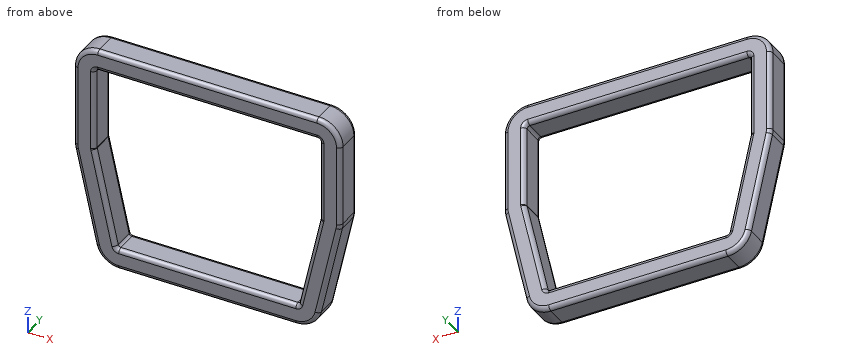
Autodesk Inventor part; units mm, degrees
ref_plane "YZ Plane" through (0, 0, 0) normal (1, 0, 0) x (0, 1, 0)
ref_plane "XZ Plane" through (0, 0, 0) normal (0, 1, 0) x (-1, 0, 0)
ref_plane "XY Plane" through (0, 0, 0) normal (0, 0, 1) x (1, 0, 0)
sketch "Sketch1" plane through (0, 0, 0) normal (0, 1, 0) x (-1, 0, 0)
  line L0 (-7.8, 0) -> (7.8, 0)
  arc A0 (8, -0.2) -> (7.8, 0) centre (7.8, -0.2) ccw
  arc A1 (-7.8, 0) -> (-8, -0.2) centre (-7.8, -0.2) ccw
  line L1 (-8, -0.2) -> (-8, -6)
  line L2 (8, -0.2) -> (8, -6)
  arc A2 (-8, -6) -> (-7.9953, -6.043) centre (-7.8, -6) ccw
  arc A3 (7.9953, -6.043) -> (8, -6) centre (7.8, -6) ccw
  line L3 (-7.9953, -6.043) -> (-6.5, -12.843)
  line L4 (7.9953, -6.043) -> (6.5, -12.843)
  arc A4 (-6.5, -12.843) -> (-6.3047, -13) centre (-6.3047, -12.8) ccw
  line L5 (-6.3047, -13) -> (6.3047, -13)
  arc A5 (6.3047, -13) -> (6.5, -12.843) centre (6.3047, -12.8) ccw
  line L6 (-9.5, -6) -> (-9.5, -0.2)
  arc A6 (-7.8, 1.5) -> (-9.5, -0.2) centre (-7.8, -0.2) ccw
  line L7 (-7.8, 1.5) -> (7.8, 1.5)
  arc A7 (9.5, -0.2) -> (7.8, 1.5) centre (7.8, -0.2) ccw
  line L8 (9.5, -0.2) -> (9.5, -6)
  arc A8 (9.4603, -6.3651) -> (9.5, -6) centre (7.8, -6) ccw
  line L9 (9.4603, -6.3651) -> (7.965, -13.1651)
  arc A9 (6.3047, -14.5) -> (7.965, -13.1651) centre (6.3047, -12.8) ccw
  line L10 (6.3047, -14.5) -> (-6.3047, -14.5)
  arc A10 (-7.965, -13.1651) -> (-6.3047, -14.5) centre (-6.3047, -12.8) ccw
  line L11 (-7.965, -13.1651) -> (-9.4603, -6.3651)
  arc A11 (-9.5, -6) -> (-9.4603, -6.3651) centre (-7.8, -6) ccw
  point P0 (0, 0)
  point P1 (0, 0)
  point P2 (0, -13)
  dimension "d0" = 0.2
  dimension "d1" = 0.2
  dimension "d2" = 16
  dimension "d3" = 6
  dimension "d4" = 0.2
  dimension "d5" = 0.2
  dimension "d6" = 0.2
  dimension "d7" = 0.2
  dimension "d8" = 13
  dimension "d9" = 13
  dimension "d10" = 1.5
extrude "Extrusion1" add sketch "Sketch1" along normal blind 2
fillet "Fillet1" radius 0.3 48 edges at (9.0021, 2, 1.0021) (9.5, 2, -3.1) (9.4901, 2, -6.1836) (8.7127, 2, -9.7651) (7.3699, 2, -14.1249) (0, 2, -14.5) (-7.3699, 2, -14.1249) (-8.7127, 2, -9.7651) (-9.4901, 2, -6.1836) (-9.5, 2, -3.1) (-9.0021, 2, 1.0021) (0, 2, 1.5) (-7.9414, 2, -0.0586) (-8, 2, -3.1) (-7.9988, 2, -6.0216) (-7.2477, 2, -9.443) (-6.43, 2, -12.9559) (0, 2, -13) (6.43, 2, -12.9559) (7.2477, 2, -9.443) (7.9988, 2, -6.0216) (8, 2, -3.1) (7.9414, 2, -0.0586) (0, 2, 0) (-9.0021, 0, 1.0021) (-9.5, 0, -3.1) (-9.4901, 0, -6.1836) (-8.7127, 0, -9.7651) (-7.3699, 0, -14.1249) (0, 0, -14.5) (7.3699, 0, -14.1249) (8.7127, 0, -9.7651) (9.4901, 0, -6.1836) (9.5, 0, -3.1) (9.0021, 0, 1.0021) (0, 0, 1.5) (7.9414, 0, -0.0586) (8, 0, -3.1) (7.9988, 0, -6.0216) (7.2477, 0, -9.443) (6.43, 0, -12.9559) (0, 0, -13) (-6.43, 0, -12.9559) (-7.2477, 0, -9.443) (-7.9988, 0, -6.0216) (-8, 0, -3.1) (-7.9414, 0, -0.0586) (0, 0, 0)
equation "\"d1\" = d0"
equation "\"d4\" = d0"
equation "\"d5\" = d4"
equation "\"d6\" = d5"
equation "\"d7\" = d6"
properties part number "y_carryage_nut_holder_a_zip_tie"
Design review of the part built by this model. Coordinates are the model's own, in mm. Round coordinates to 2 decimals unless told otherwise and drop trailing zeros. Write each loop counter-clockwise with the first axis right and the second up, starting at its lowest first coordinate (ties: lowest second). Pieces come first, ordered by that corner, then holes.
Item 1: We need section C-C on y = 0.5. Write out the cut boundary in (x, z) (3 decimals).
Item 2: We need section A-A on z = -3.75. Write out the cut boundary in (x, y).
Item 3: For probe 1 along X at (y, z) = (1.5, -4.5); probe 2 along Z at (x, y) = (-3, 1.3); probe 3 along X at (y, z) = (0.1, -3.25), list the stretches that pass through material, from the lowest coordinate up.
Item 4: We need section B-B on x = 2.25. Write out the cut boundary in (y, z), and give its area (3 significant figures).
Returned:
1. outline: (-9.5, -6) arc R1.703 ccw to (-9.46, -6.365) - (-7.965, -13.165) arc R1.7 ccw to (-6.305, -14.5) - (6.305, -14.5) arc R1.7 ccw to (7.965, -13.165) - (9.46, -6.365) arc R1.697 ccw to (9.5, -6) - (9.5, -0.2) arc R1.7 ccw to (7.8, 1.5) - (-7.8, 1.5) arc R1.7 ccw to (-9.5, -0.2) - close; hole (-8, -6) arc R0.202 ccw to (-7.995, -6.043) - (-6.5, -12.843) arc R0.2 ccw to (-6.305, -13) - (6.305, -13) arc R0.2 ccw to (6.5, -12.843) - (7.995, -6.043) arc R0.198 ccw to (8, -6) - (8, -0.2) arc R0.2 ccw to (7.8, 0) - (-7.8, 0) arc R0.2 ccw to (-8, -0.2) - close
2. outline: (-9.5, 0.3) arc R0.3 ccw to (-9.2, 0) - (-8.3, 0) arc R0.3 ccw to (-8, 0.3) - (-8, 1.7) arc R0.3 ccw to (-8.3, 2) - (-9.2, 2) arc R0.3 ccw to (-9.5, 1.7) - close; (8, 0.3) arc R0.3 ccw to (8.3, 0) - (9.2, 0) arc R0.3 ccw to (9.5, 0.3) - (9.5, 1.7) arc R0.3 ccw to (9.2, 2) - (8.3, 2) arc R0.3 ccw to (8, 1.7) - close
3. probe 1: x = -9.5 to -8, 8 to 9.5
3. probe 2: z = -14.5 to -13, 0 to 1.5
3. probe 3: x = -9.42 to -8.08, 8.08 to 9.42
4. outline: (0, -14.2) arc R0.3 ccw to (0.3, -14.5) - (1.7, -14.5) arc R0.3 ccw to (2, -14.2) - (2, -13.3) arc R0.3 ccw to (1.7, -13) - (0.3, -13) arc R0.3 ccw to (0, -13.3) - close; (0, 0.3) arc R0.3 ccw to (0.3, 0) - (1.7, 0) arc R0.3 ccw to (2, 0.3) - (2, 1.2) arc R0.3 ccw to (1.7, 1.5) - (0.3, 1.5) arc R0.3 ccw to (0, 1.2) - close
4. area: 5.85 mm2
